Part model, mm, in its own coordinate system. A direction names the side the tool comes from. Coordinates: 2 decimals unless noted, no trailing zeros. Loops run counter-clockwise (first coordinate to the right, second up) from the corner with the lowest first, then second, coordinate; pieces in that order, holes last. Notation, with made-up numbers: (54, 49) -> (99, 49) arc R6 cw to (99, 58) -> close; hole circle Ø2 at (-28, 77.5). An arc over 180 degrees is marked (long way). One line per question, with ' | ' between items. Start each with the question number.
1) Cut at A-A (y = 41). List the corners of the cut face in (x, z).
2) Cut at D-D (y = 13). List the corners of the cut face in (x, z).
3) 3-axis set-ups, long thin cutter, end or side, ignore diameter. For faces 1 (the face through (-35.556, 51.521, -26.567)), 2 (the face through (27, 43, 39.448)), 3 (the face through (38.474, 52, 70)): which of +Z, -Z, +X, -X, +Y, -Y reach the whole face in a straight line?
4) Drop flat-ended pins along their axis: pin 1 (7 mm diameter, centred on x = 38.9, z = -15.55, fed in from +Y); pin 2 (3 mm diameter, centred on x = 49.5, y = 52, fed in from +Z); pin 3 (5.5 mm diameter, centred on x = 38.9, z = 59.45, fed in from -Y); pin 4 (0.9 mm diameter, centred on x = -47.5, y = 52, fed in from -Z). Give the stop position or say it passes through.
5) Two-plate mould, pull along Z, no slides. Class faces 4 (the face through (-48.597, 26, 23)), 5 (the face through (2, 21, -28.052)), 6 (the face through (-35.97, 25.35, 56.45)), 7 (the face through (50, 52, 59.326)): released by +Z, released by -Z, zero draft, split by the parting line, or undercut.
6) Probe L1, parallel to Z at x = 37, y = 49; L2, parallel to Z at x = -35, y = 16; L3, parallel to Y at x = -12, z = 7. List the from-to ranges inside material, lowest first. Write a range as from..to.
7) Cut at C-C (z = -9.5). List the corners of the cut face in (x, y).
8) Cut at B-B (x = 26.5). List the corners of the cut face in (y, z).
from build123d import *

# Parameters (mm, degrees)
SKETCH1_W           = 100
SKETCH1_H           = 100
BOSS_EXTRUDE1_DEPTH = 50
CUT_EXTRUDE1_DEPTH  = 12
SKETCH4_R           = 3
CUT_EXTRUDE2_DEPTH  = 100
CUT_EXTRUDE3_DEPTH  = 50
BOSS_EXTRUDE4_START = 3
BOSS_EXTRUDE4_DEPTH = 3
CUT_EXTRUDE4_DEPTH  = 15
SKETCH7_R           = 1.4
BOSS_EXTRUDE5_DEPTH = 15


with BuildPart() as part:
    # Sketch1 → Boss-Extrude1 (new body)
    with BuildSketch(Plane(origin=(0, 0, 0), x_dir=(1, 0, 0), z_dir=(0, 1, 0))):
        with Locations((1.40257771, -21.948445792)):
            Rectangle(SKETCH1_W, SKETCH1_H)
    extrude(amount=BOSS_EXTRUDE1_DEPTH)

    # Sketch2 → Cut-Extrude1 (cut)
    with BuildSketch(Plane(origin=(0, 50, 0), x_dir=(1, 0, 0), z_dir=(0, 1, 0))):
        with BuildLine():
            Line((1.40257771, -4.448445792), (51.40257771, -4.448445792))
            ThreePointArc((51.40257771, -4.448445792), (68.90257771, -21.948445792), (51.40257771, -39.448445792))
            Line((51.40257771, -39.448445792), (1.40257771, -39.448445792))
            ThreePointArc((1.40257771, -39.448445792), (-16.09742229, -21.948445792), (1.40257771, -4.448445792))
        make_face()
    extrude(amount=-CUT_EXTRUDE1_DEPTH, mode=Mode.SUBTRACT)

    # Sketch4 → Cut-Extrude2 (cut)
    with BuildSketch(Plane(origin=(0, 50, 0), x_dir=(1, 0, 0), z_dir=(0, 1, 0))):
        with Locations(Location((38.90257771, 15.551554208, 0), (0, 0, 270))):
            Circle(SKETCH4_R)
        with Locations(Location((-36.09742229, 15.551554208, 0), (0, 0, 270))):
            Circle(SKETCH4_R)
        with Locations(Location((-36.09742229, -59.448445792, 0), (0, 0, 270))):
            Circle(SKETCH4_R)
        with Locations(Location((38.90257771, -59.448445792, 0), (0, 0, 270))):
            Circle(SKETCH4_R)
    extrude(amount=-CUT_EXTRUDE2_DEPTH, mode=Mode.SUBTRACT)

    # Sketch5 → Cut-Extrude3 (cut)
    with BuildSketch(Plane(origin=(0, 50, 0), x_dir=(1, 0, 0), z_dir=(0, 1, 0))):
        with BuildLine():
            Line((-48.59742229, -61.948445792), (-48.59742229, -71.948445792))
            Line((-48.59742229, -71.948445792), (-38.59742229, -71.948445792))
            ThreePointArc((-38.59742229, -71.948445792), (-45.668490101, -69.019513604), (-48.59742229, -61.948445792))
        make_face()
        with BuildLine():
            Line((-48.59742229, 28.051554208), (-38.59742229, 28.051554208))
            ThreePointArc((-38.59742229, 28.051554208), (-45.668490101, 25.12262202), (-48.59742229, 18.051554208))
            Line((-48.59742229, 18.051554208), (-48.59742229, 28.051554208))
        make_face()
        with BuildLine():
            Line((51.40257771, 28.051554208), (51.40257771, 18.051554208))
            ThreePointArc((51.40257771, 18.051554208), (48.473645522, 25.12262202), (41.40257771, 28.051554208))
            Line((41.40257771, 28.051554208), (51.40257771, 28.051554208))
        make_face()
        with BuildLine():
            Line((51.40257771, -61.948445792), (51.40257771, -71.948445792))
            Line((51.40257771, -71.948445792), (41.40257771, -71.948445792))
            ThreePointArc((41.40257771, -71.948445792), (48.473645522, -69.019513604), (51.40257771, -61.948445792))
        make_face()
    extrude(amount=-CUT_EXTRUDE3_DEPTH, mode=Mode.SUBTRACT)

    # Sketch6 → Boss-Extrude4 (add)
    with BuildSketch(Plane(origin=(0, 50, 0), x_dir=(1, 0, 0), z_dir=(0, 1, 0)).offset(BOSS_EXTRUDE4_START)):
        with BuildLine():
            ThreePointArc((38.473645522, 25.12262202), (45.544713334, 22.193689831), (48.473645522, 15.12262202))
            Line((48.473645522, 15.12262202), (51.40257771, 15.12262202))
            Line((51.40257771, 15.12262202), (51.40257771, 18.051554208))
            ThreePointArc((51.40257771, 18.051554208), (48.473645522, 25.12262202), (41.40257771, 28.051554208))
            Line((41.40257771, 28.051554208), (38.473645522, 28.051554208))
            Line((38.473645522, 28.051554208), (38.473645522, 25.12262202))
        make_face()
        with BuildLine():
            Line((-45.668490101, -59.019513604), (-48.59742229, -59.019513604))
            Line((-48.59742229, -59.019513604), (-48.59742229, -61.948445792))
            ThreePointArc((-48.59742229, -61.948445792), (-45.668490101, -69.019513604), (-38.59742229, -71.948445792))
            Line((-38.59742229, -71.948445792), (-35.668490101, -71.948445792))
            Line((-35.668490101, -71.948445792), (-35.668490101, -69.019513604))
            ThreePointArc((-35.668490101, -69.019513604), (-42.739557913, -66.090581416), (-45.668490101, -59.019513604))
        make_face()
        with BuildLine():
            Line((-35.668490101, 25.12262202), (-35.440476138, 28.051554208))
            Line((-35.440476138, 28.051554208), (-38.59742229, 28.051554208))
            ThreePointArc((-38.59742229, 28.051554208), (-45.668490101, 25.12262202), (-48.59742229, 18.051554208))
            Line((-48.59742229, 18.051554208), (-48.59742229, 15.374965532))
            Line((-48.59742229, 15.374965532), (-45.668490101, 15.12262202))
            ThreePointArc((-45.668490101, 15.12262202), (-42.739557913, 22.193689831), (-35.668490101, 25.12262202))
        make_face()
        with BuildLine():
            Line((51.40257771, -59.325952065), (48.468949193, -59.325952065))
            ThreePointArc((48.468949193, -59.325952065), (45.435528005, -66.198106245), (38.473645522, -69.019513604))
            Line((38.473645522, -69.019513604), (38.473645522, -71.948445792))
            Line((38.473645522, -71.948445792), (41.40257771, -71.948445792))
            ThreePointArc((41.40257771, -71.948445792), (48.473645522, -69.019513604), (51.40257771, -61.948445792))
            Line((51.40257771, -61.948445792), (51.40257771, -59.325952065))
        make_face()
    extrude(amount=-BOSS_EXTRUDE4_DEPTH)

    # Sketch2_2 → Cut-Extrude4 (cut)
    with BuildSketch(Plane(origin=(0, 50, 0), x_dir=(1, 0, 0), z_dir=(0, 1, 0))):
        with BuildLine():
            Line((1.40257771, -4.448445792), (51.40257771, -4.448445792))
            ThreePointArc((51.40257771, -4.448445792), (68.90257771, -21.948445792), (51.40257771, -39.448445792))
            Line((51.40257771, -39.448445792), (1.40257771, -39.448445792))
            ThreePointArc((1.40257771, -39.448445792), (-16.09742229, -21.948445792), (1.40257771, -4.448445792))
        make_face()
    extrude(amount=-CUT_EXTRUDE4_DEPTH, mode=Mode.SUBTRACT)

    # Sketch7 → Boss-Extrude5 (add)
    with BuildSketch(Plane(origin=(0, 35, 0), x_dir=(1, 0, 0), z_dir=(0, 1, 0))):
        with Locations(Location((1.40257771, -21.948445792, 0), (0, 0, 270))):
            Circle(SKETCH7_R)
    extrude(amount=BOSS_EXTRUDE5_DEPTH)


solid = part.part
Reported:
1) outline: (-48.6, -18.05) arc R10 ccw to (-38.6, -28.05) -> (41.4, -28.05) arc R10 ccw to (51.4, -18.05) -> (51.4, 4.45) -> (1.4, 4.45) arc R17.5 cw to (1.4, 39.45) -> (51.4, 39.45) -> (51.4, 61.95) arc R10 ccw to (41.4, 71.95) -> (-38.6, 71.95) arc R10 ccw to (-48.6, 61.95) -> close; circle Ø2.8 at (1.4, 21.95); hole circle Ø6 at (-36.1, -15.55); hole circle Ø6 at (-36.1, 59.45); hole circle Ø6 at (38.9, -15.55); hole circle Ø6 at (38.9, 59.45)
2) outline: (-48.6, -18.05) arc R10 ccw to (-38.6, -28.05) -> (41.4, -28.05) arc R10 ccw to (51.4, -18.05) -> (51.4, 61.95) arc R10 ccw to (41.4, 71.95) -> (-38.6, 71.95) arc R10 ccw to (-48.6, 61.95) -> close; hole circle Ø6 at (-36.1, -15.55); hole circle Ø6 at (-36.1, 59.45); hole circle Ø6 at (38.9, -15.55); hole circle Ø6 at (38.9, 59.45)
3) face 1: +Z, +Y | face 2: +X, +Y | face 3: +Z, -Z, +Y
4) pin 1: stops at y = 50 | pin 2: stops at z = 69.46 | pin 3: passes through | pin 4: stops at z = -23.4
5) face 4: zero draft | face 5: released by -Z | face 6: undercut | face 7: undercut
6) L1: z = -28.05..-17.87, -13.23..4.45, 39.45..57.13, 61.77..71.95 | L2: z = -28.05..-18.34, -12.76..56.66, 62.24..71.95 | L3: y = 0..50
7) outline: (-48.6, 0) -> (51.4, 0) -> (51.4, 50) -> (-48.6, 50) -> close
8) outline: (0, -28.05) -> (50, -28.05) -> (50, 4.45) -> (35, 4.45) -> (35, 39.45) -> (50, 39.45) -> (50, 71.95) -> (0, 71.95) -> close
